Could you check a few things on this model? Use its own coordinates, in mm. Face numbers are marked on the shaded views. A direction names the side the tool comes from. Coordinates: 2 decimals unless noted, no trailing zeros. Order: outer loops, then holes, each group sorted by start corner. A loop starts at its lowest first (then second) coordinate and runs counter-clockwise, first axis right, second up. Notation, with made-up numbers: (34.25, 54) - (62.25, 54) arc R28 cw to (62.25, 72) - close; hole circle Ø10 at (-37.5, -32.5). An arc over 180 degrees is marked (long way). One line per item, written item: value.
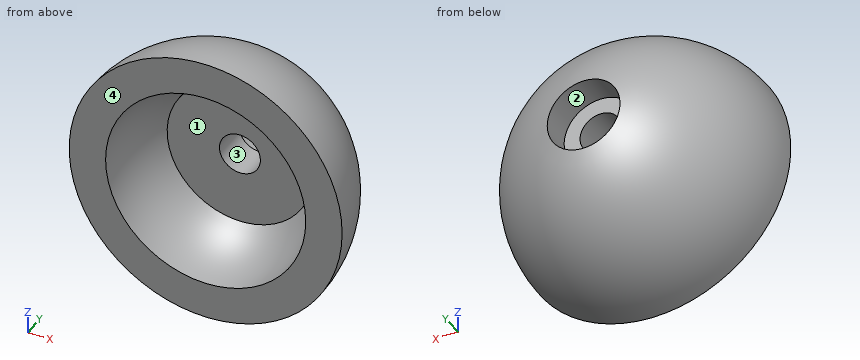
Autodesk Inventor part; units mm, degrees
ref_plane "Work Plane1" through (0, 15, 0) normal (0, 1, 0) x (-1, 0, 0)
ref_plane "YZ Plane" through (0, 0, 0) normal (1, 0, 0) x (0, 1, 0)
ref_plane "XY Plane" through (0, 0, 0) normal (0, 0, 1) x (1, 0, 0)
sketch "Sketch1" plane through (0, 0, 0) normal (0, 0, 1) x (1, 0, 0)
  line L0 (0, 0) -> (0, 15)
  line L1 (0, 0) -> (15, 0)
  arc A0 (15, 0) -> (0, 15) centre (0, 0) ccw
  line L2 (0, -3.621321) -> (0, 21.727922)
  dimension "d2" = 15
sketch "Sketch1 outline for Revolution1" plane through (0, 0, 0) normal (0, 0, 1) x (1, 0, 0)
  line L0 (0, 0) -> (0, 15)
  arc A0 (0, 15) -> (15, 0) centre (0, 0) cw
  line L1 (15, 0) -> (0, 0)
revolve "Revolution1" add sketch "Sketch1 outline for Revolution1" angle 360 about axis through (0, -10, 0) along (0, 1, 0)
ref_plane "Work Plane1" through (0, 15, 0) normal (0, 1, 0) x (-1, 0, 0)
sketch "Sketch2" plane through (0, 15, 0) normal (0, 1, 0) x (-1, 0, 0)
  point P0 (0, 0)
  point P1 (0, 0)
hole "Hole1" at (0, 15, 0) direction (0, -1, 0) diameter 4.5 end through all counterbore diameter 8 counterbore depth 4
shell "Shell1" thickness 4 removed faces 1 at (10.599241, 0, 1.286981)
sketch "Sketch3" plane through (0, 0, 0) normal (0, -1, 0) x (1, 0, 0)
  circle A0 centre (0, 0) radius 6.25
  circle A1 centre (0, 0) radius 2.25
sketch "Sketch3 outline for Extrusion1" plane through (0, 0, 0) normal (0, -1, 0) x (1, 0, 0)
  circle A0 centre (0, 0) radius 6.25
  circle A1 centre (0, 0) radius 2.25
extrude "Extrusion1" cut sketch "Sketch3 outline for Extrusion1" against normal blind 7
properties part number "Ball_Upper Half" material "Nylon 6/6"
Item 1: I want a section at A-A on z = 0. Please give me the cut outline in (x, y).
Conclusion:
outline: (-15, 0) - (-11, 0) arc R11 cw to (-8, 7.55) - (-8, 7) - (-2.25, 7) - (-2.25, 11) - (-4, 11) - (-4, 14.46) arc R15 ccw to start; (2.25, 7) - (8, 7) - (8, 7.55) arc R11 cw to (11, 0) - (15, 0) arc R15 ccw to (4, 14.46) - (4, 11) - (2.25, 11) - close
Item 2: I want a section at B-B on y = 5.5. Please give me the cut outline in (x, z).
Conclusion:
outline: circle Ø27.91 at (0, 0); hole circle Ø19.05 at (0, 0)
Item 3: I want a section at C-C on x = 7.25. Please give me the cut outline in (y, z).
Conclusion:
outline: (0, -13.13) arc R13.13 ccw to (0, 13.13) - (0, 8.27) arc R8.27 cw to (7.55, 3.38) - (7, 3.38) - (7, -3.38) - (7.55, -3.38) arc R8.27 cw to (0, -8.27) - close
Item 4: I want a section at D-D on z = 4.5. Please give me the cut outline in (x, y), then the cut area to 3 significant figures.
Conclusion:
outline: (-14.31, 0) - (-10.04, 0) arc R10.04 cw to (-6.61, 7.55) - (-6.61, 7) - (6.61, 7) - (6.61, 7.55) arc R10.04 cw to (10.04, 0) - (14.31, 0) arc R14.31 ccw to start
area: 193 mm²
Item 5: If I drill on probe 1 along X at (y, z) = (6.25, 8); probe 2 along X at (y, z) = (4, 1); probe 3 along Z at (x, y) = (0, 13.55), over which ranges is the centre line in solid material (lowest first)?
Conclusion:
probe 1: -11.04 to -4.24, 4.24 to 11.04
probe 2: -14.42 to -10.2, 10.2 to 14.42
probe 3: -6.43 to -4, 4 to 6.43
Item 6: Thinking about a two-plate mould opening in X: for the marked faces 3 and 4, which applies, pulls with the +X half, pulls with the -X half, needs draft (parallel to the pull), parting line crosses it, or undercut?
Conclusion:
face 3: undercut
face 4: needs draft
Item 7: I'm going to push flat-ended pins straight in: pin 1 Ø5 at (y, z) = (10, 7.5) entering from +X; pin 2 Ø12 at (x, z) = (3.5, 7.5) entering from +Y; pin 3 Ø1 at (y, z) = (3, 11) entering from +X; pin 4 Ø2 at (y, z) = (8.5, -8.5) entering from -X. Where does each tip first touch, or does it pass through?
Conclusion:
pin 1: x = 11.18
pin 2: y = 14.46
pin 3: x = 10.3
pin 4: x = -10.18
Item 8: For the marked faces 1 and 2, which set-ups out of +Z, -Z, +X, -X, +Y, -Y let a thin tool reach every point of the face, with its end or its side?
Conclusion:
face 1: -Y
face 2: +Y
